Input: part model. Units: mm. Frame: model coordinates. Coordinates: 2 decimals unless noted, no trailing zeros. Order: outer loops, then holes, each group sorted by start corner. A loop starts at its lowest first (then second) coordinate and runs counter-clockwise, first axis right, second up. Notation, with made-up numbers: (-27.75, 87.5) -> (-6.75, 87.5) arc R16 cw to (-6.75, 98.5) -> close; hole circle Ø6 at (70.5, 27.25). An arc over 180 degrees is marked (long way). Write each question's results on one line, items separated by ' | '.
```python
from build123d import *

# Parameters (mm, degrees)
BOSS_EXTRUDE1_OUTLINE_R        = 14.5
BOSS_EXTRUDE1_DEPTH            = 3.175
M4_CLEARANCE_HOLE1_D           = 4.5
F_3_3_3_3_DIAMETER_HOLE4_D     = 3.3
M3_CLEARANCE_HOLE2_D           = 3.4
M2X0_4_TAPPED_HOLE2_AT_2_COUNT = 2
M2X0_4_TAPPED_HOLE2_AT_2_PITCH = 86
M2X0_4_TAPPED_HOLE2_AT_3_COUNT = 2
M2X0_4_TAPPED_HOLE2_AT_3_PITCH = 103.730419839
M2X0_4_TAPPED_HOLE2_AT_4_COUNT = 2
M2X0_4_TAPPED_HOLE2_AT_4_PITCH = 58
M2X0_4_TAPPED_HOLE2_AT_5_COUNT = 2
M2X0_4_TAPPED_HOLE2_AT_5_PITCH = 97.602510214
FILLET1_R                      = 3
FILLET2_R                      = 1
FILLET3_SIZE                   = 6
FILLET3_SIZE_2                 = 9
FILLET4_R                      = 5
M3_CLEARANCE_HOLE1_D           = 3.4
M3_CLEARANCE_HOLE1_CSINK_D     = 3.45
M3_CLEARANCE_HOLE1_CSINK_ANGLE = 90
M2X0_4_TAPPED_HOLE1_D          = 1.6
CUT_EXTRUDE1_DEPTH             = 118.062568615
FILLET5_R                      = 1


with BuildPart() as part:
    # Boss-Extrude1: read off the stored shape, not the designer's step
    # Boss-Extrude1 outline → Boss-Extrude1 (new body)
    with BuildSketch(Plane(origin=(0, 0, 0), x_dir=(1, 0, 0), z_dir=(0, 1, 0))):
        with BuildLine():
            Line((33, 11.630595388), (33, 78.33262411))
            ThreePointArc((33, 78.33262411), (28.545123253, 80.063574355), (24, 81.541400528))
            Line((24, 81.541400528), (24, 45))
            Line((24, 45), (13, 45))
            Line((13, 45), (13, 24))
            Line((13, 24), (-13, 24))
            Line((-13, 24), (-13, 45))
            Line((-13, 45), (-24, 45))
            Line((-24, 45), (-24, 81.541400528))
            ThreePointArc((-24, 81.541400528), (-28.545123253, 80.063574355), (-33, 78.33262411))
            Line((-33, 78.33262411), (-33, 11.630595388))
            Line((-33, 11.630595388), (-49.185297029, 11.630595388))
            Line((-49.185297029, 11.630595388), (-52.624325057, 21.384301413))
            Line((-52.624325057, 21.384301413), (-58.624325057, 21.384301413))
            Line((-58.624325057, 21.384301413), (-58.624325057, 26.630595388))
            Line((-58.624325057, 26.630595388), (-68.191318528, 26.630595388))
            Line((-68.191318528, 26.630595388), (-77.073860284, 35.841596796))
            ThreePointArc((-77.073860284, 35.841596796), (-84.367778143, 10.347850562), (-83.451078309, -16.152941807))
            Line((-83.451078309, -16.152941807), (-75.073268231, -10.906716078))
            Line((-75.073268231, -10.906716078), (-66.121429656, -10.906716078))
            Line((-66.121429656, -10.906716078), (-53.091566877, -24.906716078))
            Line((-53.091566877, -24.906716078), (-34.205297029, -24.906716078))
            Line((-34.205297029, -24.906716078), (-34.205297029, -39))
            Line((-34.205297029, -39), (60.196181169, -39))
            Line((60.196181169, -39), (60.196181169, -17.27312839))
            Line((60.196181169, -17.27312839), (66.121429656, -10.906716078))
            Line((66.121429656, -10.906716078), (75.073268231, -10.906716078))
            Line((75.073268231, -10.906716078), (83.451078309, -16.152941807))
            ThreePointArc((83.451078309, -16.152941807), (84.367778143, 10.347850562), (77.073860284, 35.841596796))
            Line((77.073860284, 35.841596796), (55.268726082, 28.884301413))
            Line((55.268726082, 28.884301413), (49.185297029, 11.630595388))
            Line((49.185297029, 11.630595388), (33, 11.630595388))
        make_face()
        with Locations((-68.685297029, 8.424)):
            Circle(BOSS_EXTRUDE1_OUTLINE_R, mode=Mode.SUBTRACT)
        Polygon((-49.185297029, -18.906716078), (-49.185297029, 7.630595388), (-29, 7.630595388), (-29, 20.630595388), (-21.3, 20.630595388), (-21.3, -18.906716078), align=None, mode=Mode.SUBTRACT)
        Polygon((29, 20.630595388), (29, 7.630595388), (49.185297029, 7.630595388), (49.185297029, -27.138060345), (21.3, -27.138060345), (21.3, 20.630595388), align=None, mode=Mode.SUBTRACT)
        with Locations((68.685297029, 8.424)):
            Circle(BOSS_EXTRUDE1_OUTLINE_R, mode=Mode.SUBTRACT)
    extrude(amount=BOSS_EXTRUDE1_DEPTH)

    # M4 Clearance Hole1 (through all)
    with Locations(Plane(origin=(0, 3.175, 0), x_dir=(1, 0, 0), z_dir=(0, 1, 0))):
        with Locations((-78.54120923, -8.5016735), (78.54120923, -8.5016735)):
            Hole(M4_CLEARANCE_HOLE1_D / 2)

    # Ø3.3 (3.3) Diameter Hole4 (through all)
    with Locations(Plane(origin=(0, 3.175, 0), x_dir=(1, 0, 0), z_dir=(0, 1, 0))):
        with Locations((17.5, 15.4), (-17.5, -18), (-17.5, 15.4), (17.5, -18)):
            Hole(F_3_3_3_3_DIAMETER_HOLE4_D / 2)

    # M3 Clearance Hole2 (through all)
    with Locations(Plane(origin=(0, 3.175, 0), x_dir=(1, 0, 0), z_dir=(0, 1, 0))):
        with Locations((28.19, 74.751400528), (-28.19, 74.751400528)):
            Hole(M3_CLEARANCE_HOLE2_D / 2)

    # Sketch15 → M2x0.4 Tapped Hole2 (revolve, cut)
    with BuildSketch(Plane(origin=(-29.558455866, 3.175, -25.380595388), x_dir=(0, 0, 1), z_dir=(1, 0, 0))):
        Polygon((0, 0), (0, 3.175), (1.5, 3.175), (0.8, 2.475), (0.8, 0), align=None)
    m2x0_4_tapped_hole2 = revolve(axis=Axis((-29.558455866, 9.525, -25.380595388), (0, -1, 0)), mode=Mode.SUBTRACT)

    # M2x0.4 Tapped Hole2 at 2: M2x0.4 Tapped Hole2 ×2
    with Locations(*[(i * M2X0_4_TAPPED_HOLE2_AT_2_PITCH, 0, 0) for i in range(1, M2X0_4_TAPPED_HOLE2_AT_2_COUNT)]):
        add(m2x0_4_tapped_hole2, mode=Mode.SUBTRACT)

    # M2x0.4 Tapped Hole2 at 3: M2x0.4 Tapped Hole2 ×2
    with Locations(*[Vector(0.8290721288256765, 0, 0.5591416682777818) * (i * M2X0_4_TAPPED_HOLE2_AT_3_PITCH) for i in range(1, M2X0_4_TAPPED_HOLE2_AT_3_COUNT)]):
        add(m2x0_4_tapped_hole2, mode=Mode.SUBTRACT)

    # M2x0.4 Tapped Hole2 at 4: M2x0.4 Tapped Hole2 ×2
    with Locations(*[(0, 0, i * M2X0_4_TAPPED_HOLE2_AT_4_PITCH) for i in range(1, M2X0_4_TAPPED_HOLE2_AT_4_COUNT)]):
        add(m2x0_4_tapped_hole2, mode=Mode.SUBTRACT)

    # M2x0.4 Tapped Hole2 at 5: M2x0.4 Tapped Hole2 ×2
    with Locations(*[Vector(0.8042825930213097, 0, 0.59424701140428) * (i * M2X0_4_TAPPED_HOLE2_AT_5_PITCH) for i in range(1, M2X0_4_TAPPED_HOLE2_AT_5_COUNT)]):
        add(m2x0_4_tapped_hole2, mode=Mode.SUBTRACT)

    # Fillet1
    fillet1_edges = [part.edges().sort_by_distance(p)[0] for p in [
        (75.073268231, 1.5875, 10.906716078),
        (66.121429656, 1.5875, 10.906716078),
        (-66.121429656, 1.5875, 10.906716078),
        (-75.073268231, 1.5875, 10.906716078),
        (-68.191318528, 1.5875, -26.630595388),
        (-33, 1.5875, -78.33262411),
        (-24, 1.5875, -81.541400528),
        (24, 1.5875, -81.541400528),
        (33, 1.5875, -78.33262411),
    ]]
    fillet(fillet1_edges, radius=FILLET1_R)

    # Fillet2
    fillet2_edges = [part.edges().sort_by_distance(p)[0] for p in [
        (33, 1.5875, -11.630595388),
        (49.185297029, 1.5875, -11.630595388),
        (55.268726082, 1.5875, -28.884301413),
        (77.073860284, 1.5875, -35.841596796),
        (83.451078309, 1.5875, 16.152941807),
        (60.196181169, 1.5875, 17.27312839),
        (60.196181169, 1.5875, 39),
        (-34.205297029, 1.5875, 39),
        (-34.205297029, 1.5875, 24.906716078),
        (-53.091566877, 1.5875, 24.906716078),
        (-83.451078309, 1.5875, 16.152941807),
        (-77.073860284, 1.5875, -35.841596796),
        (-58.624325057, 1.5875, -26.630595388),
        (-58.624325057, 1.5875, -21.384301413),
        (-52.624325057, 1.5875, -21.384301413),
        (-49.185297029, 1.5875, -11.630595388),
        (-33, 1.5875, -11.630595388),
        (-24, 1.5875, -45),
        (-13, 1.5875, -45),
        (13, 1.5875, -45),
        (24, 1.5875, -45),
        (-49.185297029, 1.5875, -7.630595388),
        (-21.3, 1.5875, -20.630595388),
        (-29, 1.5875, -20.630595388),
        (-29, 1.5875, -7.630595388),
        (29, 1.5875, -20.630595388),
        (21.3, 1.5875, -20.630595388),
        (49.185297029, 1.5875, -7.630595388),
        (29, 1.5875, -7.630595388),
    ]]
    fillet(fillet2_edges, radius=FILLET2_R)

    # Fillet3
    # a fillet whose section is not a circle: 9, 6 mm, written as the material it adds along each edge
    with BuildSketch(Plane(origin=(13, 0, -24), x_dir=(0, 0, -1), z_dir=(0, 1, 0))) as fillet3_piece_1:
        with BuildLine():
            Bezier((FILLET3_SIZE, 0), (0, 0), (0, FILLET3_SIZE_2), weights=[1, 0.666666667, 1])
            Line((0, FILLET3_SIZE_2), (0, 0))
            Line((0, 0), (FILLET3_SIZE, 0))
        make_face()
    extrude(amount=3.175)
    with BuildSketch(Plane(origin=(-13, 0, -24), x_dir=(1, 0, 0), z_dir=(0, 1, 0))) as fillet3_piece_2:
        with BuildLine():
            Bezier((FILLET3_SIZE_2, 0), (0, 0), (0, FILLET3_SIZE), weights=[1, 0.666666667, 1])
            Line((0, FILLET3_SIZE), (0, 0))
            Line((0, 0), (FILLET3_SIZE_2, 0))
        make_face()
    extrude(amount=3.175)

    # Fillet4
    fillet4_edges = [part.edges().sort_by_distance(p)[0] for p in [
        (-49.185297029, 1.5875, 18.906716078),
        (-21.3, 1.5875, 18.906716078),
        (21.3, 1.5875, 27.138060345),
        (49.185297029, 1.5875, 27.138060345),
    ]]
    fillet(fillet4_edges, radius=FILLET4_R)

    # M3 Clearance Hole1 (through all)
    with Locations(Plane(origin=(0, 3.175, 0), x_dir=(1, 0, 0), z_dir=(0, 1, 0))):
        with Locations((75, 29), (-75, 29)):
            CounterSinkHole(M3_CLEARANCE_HOLE1_D / 2, M3_CLEARANCE_HOLE1_CSINK_D / 2, counter_sink_angle=M3_CLEARANCE_HOLE1_CSINK_ANGLE)

    # M2x0.4 Tapped Hole1 (through all)
    with Locations(Plane(origin=(0, 3.175, 0), x_dir=(1, 0, 0), z_dir=(0, 1, 0))):
        with Locations((-20, -32), (20, -32)):
            Hole(M2X0_4_TAPPED_HOLE1_D / 2)

    # Sketch32 → Cut-Extrude1 (cut, through all)
    with BuildSketch(Plane(origin=(0, 3.175, 0), x_dir=(1, 0, 0), z_dir=(0, 1, 0))):
        with BuildLine():
            Line((49.196181169, -39), (60.196181169, -21.396320181))
            Line((60.196181169, -21.396320181), (60.196181169, -38))
            ThreePointArc((60.196181169, -38), (59.90328795, -38.707106781), (59.196181169, -39))
            Line((59.196181169, -39), (49.196181169, -39))
        make_face()
    extrude(amount=-CUT_EXTRUDE1_DEPTH, mode=Mode.SUBTRACT)

    # Fillet5
    fillet5_edges = [part.edges().sort_by_distance(p)[0] for p in [
        (49.196181169, 1.5875, 39),
        (60.196181169, 1.5875, 21.396320181),
    ]]
    fillet(fillet5_edges, radius=FILLET5_R)


solid = part.part
```
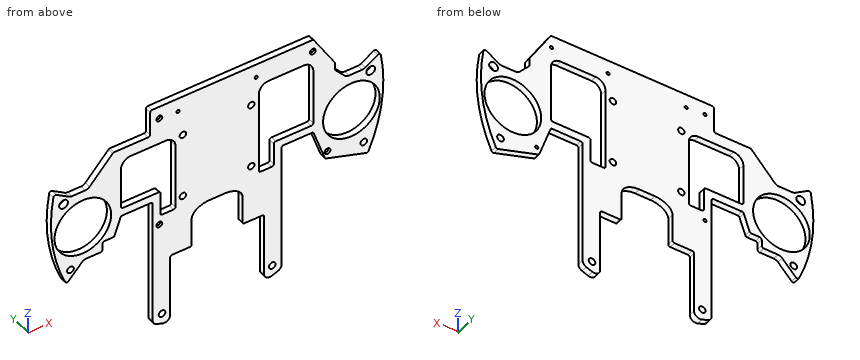
(1) Pin query (flat end, axial travel): P1, Ø1, axis at y = 2.5, z = -12, coming from the +X side; P2, Ø1.6, axis at x = 18, y = 2, coming from the -Z side; P3, Ø1.6, axis at y = 1, z = 20, coming from the +X side; P4, Ø10, axis at x = 59, z = -26, coming from the -Y side. Return the tip coordinate at first contact, or that it passes through.
Return value:
P1: x = 84.22 | P2: z = -45 | P3: x = 60.2 | P4: y = 0
(2) Cut plane B-B, the plane x = 63. Return loops of the section in (y, z) (3 decimals), plus the area to 3 significant figures.
Return value:
outline: (0, -31.351) -> (3.175, -31.351) -> (3.175, -21.763) -> (0, -21.763) -> close; (0, 4.915) -> (3.175, 4.915) -> (3.175, 14.261) -> (0, 14.261) -> close | area: 60.1 mm2
(3) Line query: line 1 along X through (y, z) = (1.15, -5); line 2 along X through (y, z) = (2.25, -51); line 3 along X through (y, z) = (0.85, -2). Output: solid intervals per line, ascending. Write a range as from..to.
Return value:
line 1: -84.85..-82.78, -54.6..-49.19, -21.3..21.3, 49.19..54.6, 82.78..84.85 | line 2: -33..-24, 24..33 | line 3: -84.98..-81.68, -55.69..-49.19, -21.3..21.3, 49.19..55.69, 81.68..84.98
(4) Cut plane C-C, the plane y = 2.5. Count the separate pieces of the cut face and the enclosed holes in it, plus the area to 3 significant figures.
Return value:
separate pieces: 1 | enclosed holes: 20 | area: 6,880 mm2
(5) Cut plane A-A, the plane z = -40. Return loops of the section in (x, y) (3 decimals), plus the area to 3 significant figures.
Return value:
outline: (-33, 0) -> (-13, 0) -> (-13, 3.175) -> (-33, 3.175) -> close; (13, 0) -> (33, 0) -> (33, 3.175) -> (13, 3.175) -> close | area: 127 mm2
